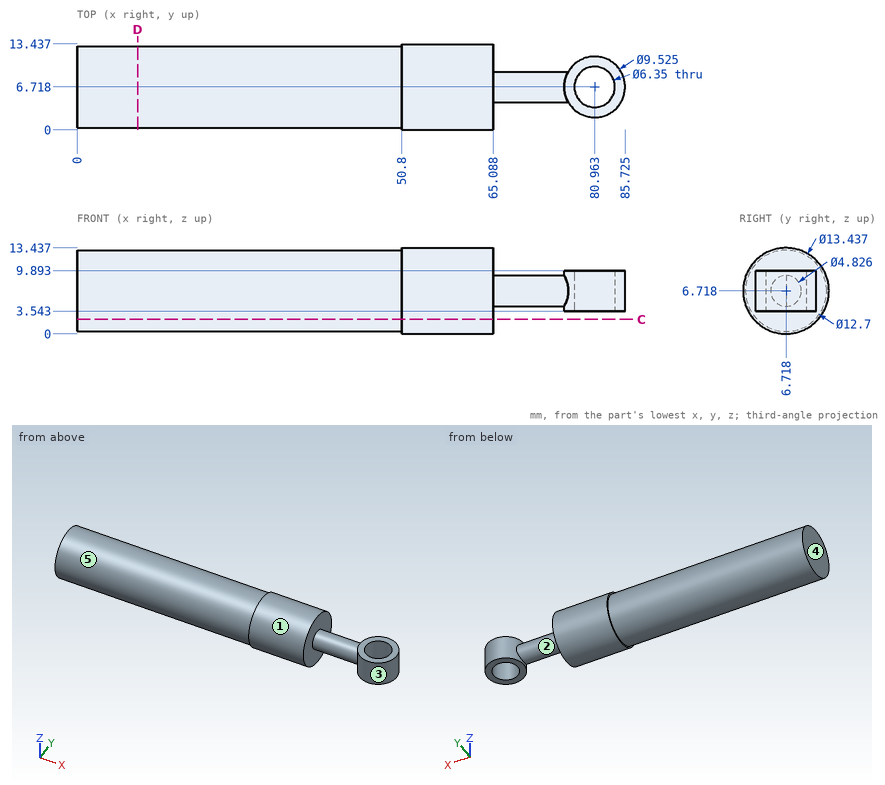
Here's the drawing with two shaded views (mm, measured from the low corner). I have some questions. A direction names the side the tool comes from. Give positions to 0.01 mm unless a question says otherwise; leave off trailing zeros. Order: outer loops, then holes, each group sorted by start corner. A loop starts at its lowest first (then second) coordinate and runs counter-clockwise, first axis right, second up.
Q1. Suppose I cut it at D-D, the plane x = 9.5. Write out the boundary of the cut face in (y, z), and give its area (3 significant figures).
Q2. We'd pull the mould along X, two halves only. Please class the marked faces 3, 4 and 5: +X half, -X half, draft (parallel to the pull), parting line (faces both ways), or undercut.
Q3. Suppose I cut it at C-C, the plane z = 2.25. Write out the boundary of the cut face in (x, y) (1 decimal).
Q4. If I drill on line 1 along X through (y, z) = (5, 2); line 2 along X through (y, z) = (5, 7) (1 decimal); line 3 along Y through (x, z) = (10, 6.75), over which ranges is the centre line in solid material (lowest first)?
Q5. For the marked faces 1 and 2, which set-ups out of +Z, -Z, +X, -X, +Y, -Y let a thin tool reach every point of the face, with its end or its side?
Q6. I'm going to push flat-ended pins straight in: P1, Ø2, axis at y = 7, z = 2.5, coming from the +X side; P2, Ø8, axis at x = 23.5, z = 11.5, coming from the +Y side; P3, Ø6, axis at x = 75, y = 6.5, coming from the +Z side. Where does each tip first touch, or does it pass through?
Solution:
1. outline: circle Ø12.7 at (6.72, 6.72)
1. area: 127 mm2
2. face 3: undercut
2. face 4: -X half
2. face 5: draft
3. outline: (0, 2.2) - (50.8, 2.2) - (50.8, 1.7) - (65.1, 1.7) - (65.1, 11.7) - (50.8, 11.7) - (50.8, 11.2) - (0, 11.2) - close
4. line 1: x = 0 to 65.09
4. line 2: x = 0 to 78.3, 83.6 to 85.4
4. line 3: y = 0.37 to 13.07
5. face 1: +X, -X
5. face 2: none
6. P1: stops at x = 65.09
6. P2: stops at y = 13.02
6. P3: stops at z = 9.89
